Could you check a few things on this model? Use its own coordinates, in mm. Face numbers are marked on the shaded views. A direction names the side the tool comes from. Coordinates: 2 decimals unless noted, no trailing zeros. Loops run counter-clockwise (first coordinate to the right, second up) from the corner with the lowest first, then second, coordinate; pieces in that order, holes last. Notation, with made-up numbers: M -4.75,58.25 L 53.25,58.25 A19 cw 53.25,87.25 Z; hole C 49,-6 d10. An arc over 180 degrees is marked long. Write each question's results on one line, items separated by ' | '.
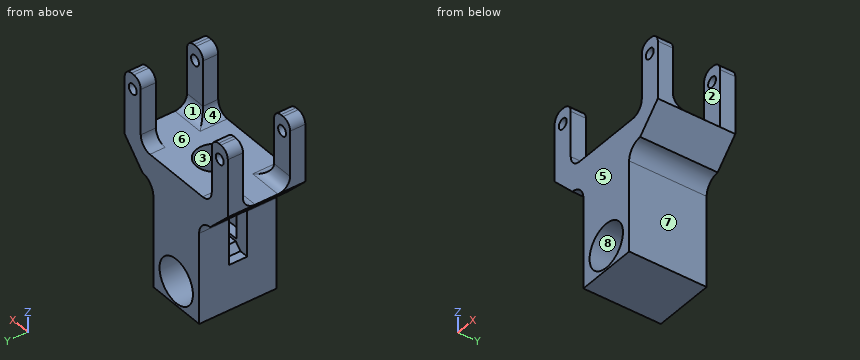
```python
from build123d import *

# Parameters (mm, degrees)
BOSS_EXTRU_1_DEPTH                    = 25.5
ENL_V_MAT_EXTRU_1_REACH               = 52.178
ESQUISSE2_W                           = 19.17973925
ESQUISSE2_H                           = 6
ESQUISSE3_W                           = 5
ESQUISSE3_H                           = 2.04072335
BOSS_EXTRU_2_DEPTH                    = 6
ESQUISSE4_W                           = 7
ESQUISSE4_H                           = 5
BOSS_EXTRU_3_DEPTH                    = 22
ESQUISSE5_W                           = 7
ESQUISSE5_H                           = 5
BOSS_EXTRU_4_DEPTH                    = 22
ESQUISSE6_W                           = 7
ESQUISSE6_H                           = 5
BOSS_EXTRU_5_DEPTH                    = 22
ESQUISSE7_W                           = 7
ESQUISSE7_H                           = 5
BOSS_EXTRU_6_DEPTH                    = 22
D_POUILLE1_ANGLE                      = 45
D_GAGEMENT_M121_D                     = 14.566399692
D_GAGEMENT_M31_D                      = 3.44556842
D_GAGEMENT_M31_DEPTH                  = 5
D_GAGEMENT_M32_D                      = 3.44556842
D_GAGEMENT_M33_D                      = 3.44556842
D_GAGEMENT_M33_DEPTH                  = 25.5
DIAM_TRE_DU_PER_AGE_12_2_12_2_1_D     = 12.2
DIAM_TRE_DU_PER_AGE_12_2_12_2_1_DEPTH = 25
CONG_1_R                              = 3
CONG_2_R                              = 4


with BuildPart() as part:
    # Esquisse1 → Boss.-Extru.1 (new body)
    with BuildSketch(Plane(origin=(0, 12.75, 0), x_dir=(1, 0, 0), z_dir=(0, 1, 0))):
        with BuildLine():
            Line((-22.5, 0), (22.5, 0))
            Line((22.5, 0), (22.5, 0.009618943))
            Line((22.5, 0.009618943), (14.807692308, 8.003699594))
            ThreePointArc((14.807692308, 8.003699594), (11.397116539, 9.533123774), (10, 13))
            Line((10, 13), (10, 43))
            Line((10, 43), (-10, 43))
            Line((-10, 43), (-10, 13))
            ThreePointArc((-10, 13), (-11.397116539, 9.533123774), (-14.807692308, 8.003699594))
            Line((-14.807692308, 8.003699594), (-22.5, 0.009618943))
            Line((-22.5, 0.009618943), (-22.5, 0))
        make_face()
    extrude(amount=-BOSS_EXTRU_1_DEPTH)

    # Esquisse2 → Enlèv. mat.-Extru.1 (cut, up to next)
    with BuildSketch(Plane(origin=(0, 0, 0), x_dir=(0, 0, -1), z_dir=(1, 0, 0)), mode=Mode.PRIVATE) as enl_v_mat_extru_1_sk1:
        with Locations((18.410130375, -0.071525989)):
            Rectangle(ESQUISSE2_W, ESQUISSE2_H)
    enl_v_mat_extru_1_tool1 = extrude(enl_v_mat_extru_1_sk1.sketch, amount=-ENL_V_MAT_EXTRU_1_REACH, mode=Mode.PRIVATE) & part.part
    add(enl_v_mat_extru_1_tool1.solids().sort_by_distance((0, -0.071526, -18.41013))[0], mode=Mode.SUBTRACT)

    # Esquisse3 → Boss.-Extru.2 (add)
    with BuildSketch(Plane(origin=(0, -3.071525989, 0), x_dir=(-1, 0, 0), z_dir=(0, 1, 0))):
        with Locations((2.5, -26.979638325)):
            Rectangle(ESQUISSE3_W, ESQUISSE3_H)
    extrude(amount=BOSS_EXTRU_2_DEPTH)

    # Esquisse4 → Boss.-Extru.3 (add)
    with BuildSketch(Plane.XY):
        with Locations((19, 10.25)):
            Rectangle(ESQUISSE4_W, ESQUISSE4_H)
    extrude(amount=BOSS_EXTRU_3_DEPTH)

    # Esquisse5 → Boss.-Extru.4 (add)
    with BuildSketch(Plane.XY):
        with Locations((-19, 10.25)):
            Rectangle(ESQUISSE5_W, ESQUISSE5_H)
    extrude(amount=BOSS_EXTRU_4_DEPTH)

    # Esquisse6 → Boss.-Extru.5 (add)
    with BuildSketch(Plane.XY):
        with Locations((19, -10.25)):
            Rectangle(ESQUISSE6_W, ESQUISSE6_H)
    extrude(amount=BOSS_EXTRU_5_DEPTH)

    # Esquisse7 → Boss.-Extru.6 (add)
    with BuildSketch(Plane.XY):
        with Locations((-19, -10.25)):
            Rectangle(ESQUISSE7_W, ESQUISSE7_H)
    extrude(amount=BOSS_EXTRU_6_DEPTH)

    # Dépouille1
    d_pouille1_faces = [part.faces().sort_by_distance(p)[0] for p in [
        (-5, -0.071525989, -26.979638325),
    ]]
    draft(d_pouille1_faces, Plane(origin=(0, 2.928474011, -25.95927665), x_dir=(0, 1, 0), z_dir=(0, 0, 1)), D_POUILLE1_ANGLE)

    # Dégagement M121 (through all)
    with Locations(Plane(origin=(0, -12.75, 0), x_dir=(-1, 0, 0), z_dir=(0, -1, 0))):
        with Locations((0, 34.962736357)):
            Hole(D_GAGEMENT_M121_D / 2)

    # Dégagement M31
    with Locations(Plane(origin=(0, 12.75, 0), x_dir=(1, 0, 0), z_dir=(0, 1, 0))):
        with Locations((-19, -17), (19, -17)):
            Hole(D_GAGEMENT_M31_D / 2, depth=D_GAGEMENT_M31_DEPTH)

    # Dégagement M32 (through all)
    with Locations(Plane(origin=(0, -7.75, 0), x_dir=(1, 0, 0), z_dir=(0, 1, 0))):
        with Locations((19, -17)):
            Hole(D_GAGEMENT_M32_D / 2)

    # Dégagement M33
    with Locations(Plane(origin=(0, -12.75, 0), x_dir=(-1, 0, 0), z_dir=(0, -1, 0))):
        with Locations((19, -17)):
            Hole(D_GAGEMENT_M33_D / 2, depth=D_GAGEMENT_M33_DEPTH)

    # Diamètre du perçage Ø12.2 (12.2)1
    with Locations(Plane.XY):
        with Locations((0, 0)):
            Hole(DIAM_TRE_DU_PER_AGE_12_2_12_2_1_D / 2, depth=DIAM_TRE_DU_PER_AGE_12_2_12_2_1_DEPTH)

    # Congé1
    cong_1_edges = [part.edges().sort_by_distance(p)[0] for p in [
        (15.5, -10.25, 22),
        (22.5, -10.25, 22),
        (-15.5, -10.25, 22),
        (-22.5, -10.25, 22),
        (15.5, 10.25, 22),
        (22.5, 10.25, 22),
        (-22.5, 10.25, 22),
        (-15.5, 10.25, 22),
    ]]
    fillet(cong_1_edges, radius=CONG_1_R)

    # Congé2
    cong_2_edges = [part.edges().sort_by_distance(p)[0] for p in [
        (-19, -7.75, 0),
        (-15.5, -10.25, 0),
        (15.5, 10.25, 0),
        (-19, 7.75, 0),
        (-15.5, 10.25, 0),
        (19, -7.75, 0),
        (15.5, -10.25, 0),
    ]]
    fillet(cong_2_edges, radius=CONG_2_R)


solid = part.part
```
(1) Imagine slicing it at A-A, the plane y = 0. State how many separate pieces and enclosed holes the cut face has, and give its area (3 significant figures).
Reported:
separate pieces: 2 | enclosed holes: 1 | area: 454 mm2
(2) Please list where these lines run through material, in increasing order: probe 1 along X at (y, z) = (10.5, 17); probe 2 along X at (y, z) = (-5.25, -35); probe 3 along Z at (x, y) = (-9.5, -0.75). Write a range as from..to.
Reported:
probe 1: x = -22.5..-20.72, -17.28..-15.5, 15.5..17.28, 20.72..22.5 | probe 2: x = -10..-7.28, 7.28..10 | probe 3: z = -43..-28, -8.82..0
(3) If we mould it in two halves opening along X, with no side actions, what happens to the marked faces 5, 6, 7 and 8? For each: released by +X, released by -X, zero draft, split by the parting line, or undercut.
Reported:
face 5: zero draft | face 6: undercut | face 7: released by +X | face 8: undercut
(4) Imagine slicing it at D-D, the plane y = -10. List the corners of the cut face in (x, z) for me, and give its area (3 significant figures).
Reported:
outline: M -22.5,-0.01 L -14.81,-8 A5 cw -10,-13 L -10,-43 L 10,-43 L 10,-13 A5 cw 14.81,-8 L 22.5,-0.01 L 22.5,19 A3 ccw 19.5,22 L 18.5,22 A3 ccw 15.5,19 L 15.5,4 A4 cw 11.5,0 L -11.5,0 A4 cw -15.5,4 L -15.5,19 A3 ccw -18.5,22 L -19.5,22 A3 ccw -22.5,19 Z; hole C -19,17 d3.45; hole C 0,-34.96 d14.57; hole C 19,17 d3.45 | area: 1,130 mm2
(5) Which directions (+Z, -Z, +X, -X, +Y, -Y) give clear straight access to the entire face, cutting with the end or side of a thin tool? Please do the marked faces 1, 2, 3 and 4.
Reported:
face 1: +Z, +X, -X | face 2: +Z, +X | face 3: +Z | face 4: +Z, +Y, -Y
(6) Imagine slicing it at C-C, the plane x = 5. List the corners of the cut face in (y, z) for me.
Reported:
outline: M -12.75,-43 L 12.75,-43 L 12.75,-40.26 L -12.75,-40.26 Z; M -12.75,-29.67 L 12.75,-29.67 L 12.75,0 L 3.49,0 L 3.49,-25 L -3.49,-25 L -3.49,0 L -12.75,0 Z
(7) Will these pins go through, and if not, where does the flat tip stop? P1, Ø3.5, axis at x = -8, y = -1, coming from the +Z side; P2, Ø2, axis at x = -19, z = 17, coming from the +Y side; P3, Ø3.5, axis at x = -0.5, y = -0.5, coming from the +Z side; P4, Ø4, axis at y = 4.5, z = -23, coming from the -X side.
Reported:
P1: stops at z = 0 | P2: passes through | P3: stops at z = -25 | P4: stops at x = -10
